Input: part model. Units: mm. Frame: model coordinates. A direction names the side the tool comes from. Coordinates: 2 decimals unless noted, no trailing zeros. Loops run counter-clockwise (first coordinate to the right, second up) from the corner with the lowest first, then second, coordinate; pieces in that order, holes last.
(1) Section B-B, the plane z = 0. Return loops of the section in (x, y).
(2) Line query: L1, parallel to X at y = -1, z = 3.25; L2, parallel to Z at x = 4.25, y = -4.75; L3, parallel to Y at x = 2.5, z = 0. Output: solid intervals per line, ascending.
(3) Section A-A, the plane y = 0. Return loops of the section in (x, z).
(4) Mould query, pull axis Y, two halves, no side actions, for faces 1 (the face through (2.13, 6.75, 0.02)), 2 (the face through (3.8, 0, -2.3)), 3 (the face through (0, -2, -1)). Classes: released by +Y, released by -Y, zero draft, split by the parting line, or undercut.
(5) Contact query for flat-ended pins moving along their axis: P1, Ø5.5, axis at x = 5.5, y = -7, coming from the -Z side; P2, Ø1, axis at y = -0.5, z = -2, coming from the +X side; P3, Ø5.5, axis at x = 4.5, y = -7, coming from the +Z side. Output: stop coordinate, or through.
(6) Section C-C, the plane x = 4. Return loops of the section in (y, z), then the cut area to 3 significant figures.
(7) Set-up query: faces 4 (the face through (5.431, 3.767, 0.019)), 5 (the face through (2.13, -6.75, 0.02)). Return all of +Z, -Z, +X, -X, +Y, -Y with unobstructed straight access to the full face (end or side cutting, diameter ignored); none if empty.
(8) Section D-D, the plane z = -1. Return loops of the section in (x, y).
```python
from build123d import *

# Parameters (mm, degrees)
BOSS_EXTRUDE1_DEPTH = 1.333333333


with BuildPart() as part:
    # Sketch2 → Revolve1 (revolve)
    with BuildSketch(Plane(origin=(0, 0, 0), x_dir=(1, 0, 0), z_dir=(0, 1, 0)), mode=Mode.PRIVATE) as revolve1_sk:
        Polygon((0, 2), (0, 4.5), (3.8, 3.481793069), (3.8, 2), align=None)
    revolve(revolve1_sk.sketch.rotate(Axis((0, 0, 0), (1, 0, 0)), 180), axis=Axis((0, 0, 0), (1, 0, 0)))

    # Sketch3 → Boss-Extrude1 (add, symmetric)
    with BuildSketch(Plane.XY):
        with BuildLine():
            Line((0, 4.5), (4.321922287, 9.063002054))
            ThreePointArc((4.321922287, 9.063002054), (9.142888967, 8.419555533), (7.017244249, 4.04492667))
            Line((7.017244249, 4.04492667), (3.8, 3.481793069))
            Line((3.8, 3.481793069), (3.8, 2))
            Line((3.8, 2), (0, 2))
            Line((0, 2), (0, 4.5))
        make_face()
    boss_extrude1 = extrude(amount=BOSS_EXTRUDE1_DEPTH, both=True)

    # Mirror1: Boss-Extrude1 across plane
    add(boss_extrude1.mirror(Plane.ZX))


solid = part.part
```
Report:
1. outline: (0, -4.5) - (4.32, -9.06) arc R3 ccw (long way) to (7.02, -4.04) - (3.8, -3.48) - (3.8, -2) - (0, -2) - close; (0, 2) - (3.8, 2) - (3.8, 3.48) - (7.02, 4.04) arc R3 ccw (long way) to (4.32, 9.06) - (0, 4.5) - close
2. L1: x = 0 to 3.8
2. L2: z = -1.33 to 1.33
2. L3: y = -7.14 to -2, 2 to 7.14
3. outline: (0, -4.5) - (3.8, -3.48) - (3.8, -2) - (0, -2) - close; (0, 2) - (3.8, 2) - (3.8, 3.48) - (0, 4.5) - close
4. face 1: released by +Y
4. face 2: undercut
4. face 3: zero draft
5. P1: stops at z = -1.33
5. P2: stops at x = 3.8
5. P3: stops at z = 1.33
6. outline: (-8.72, -1.33) - (-3.52, -1.33) - (-3.52, 1.33) - (-8.72, 1.33) - close; (3.52, -1.33) - (8.72, -1.33) - (8.72, 1.33) - (3.52, 1.33) - close
6. area: 27.8 mm2
7. face 4: +Z, -Z, +X
7. face 5: +Z, -Z, -X, -Y
8. outline: (0, -4.5) - (4.32, -9.06) arc R3 ccw (long way) to (7.02, -4.04) - (3.8, -3.48) - (3.8, -1.73) - (0, -1.73) - close; (0, 1.73) - (3.8, 1.73) - (3.8, 3.48) - (7.02, 4.04) arc R3 ccw (long way) to (4.32, 9.06) - (0, 4.5) - close
